Study the drawing (mm; zero at the part's minimum x, y, z) and answer. A direction names the side the tool comes from. Coordinates: 2 decimals unless noted, no trailing zeros. Order: outer loops, then holes, each group sorted by start corner. A loop starts at its lowest first (then second) coordinate and runs counter-clockwise, first axis right, second up. Notation, with made-up numbers: (-30, -18) -> (22, -18) arc R28 cw to (22, 11) -> close; hole circle Ø10 at (19.5, 55). An arc over 180 degrees is marked (long way). Answer as CSV lines item,"result". Start each with the question number.
Item 1: Each of these flat-tipped pins is pushed along its axis until it touches: pin 1 Ø4 at (x, y) = (15.5, 8) entering from -Z; pin 2 Ø1.5 at (x, y) = (18, 8) entering from +Z; pin 3 Ø5 at (x, y) = (51.5, 6.5) entering from -Z; pin 4 Ø5.5 at (x, y) = (83, 7) entering from +Z. Where does it stop, or does it pass through?
Item 2: Section B-B (y = 2.75) is taken. Write down the section's boundary in (x, z).
Item 3: For a pull along X with two mould halves and no side action, classify the marked faces 4 and 5 as pulls with the +X half, pulls with the -X half, needs draft (parallel to the pull), parting line crosses it, or undercut.
Item 4: Section A-A (z = 9) is taken. Write down the section's boundary in (x, y), then the cut area to 3 significant figures.
Item 5: Section D-D (z = 72.5) is taken. Write down the section's boundary in (x, y).
Item 6: Straight lines are drawn through the part: L1, parallel to X at y = 2, z = 95; L2, parallel to X at y = 9.75, z = 7.5; L3, parallel to Z at x = 62, y = 7.75. For each, find the intervals that lie inside material, in ascending order.
Item 7: Section C-C (x = 13) is taken. Write down the section's boundary in (y, z).
Item 8: Which of the six approach directions +Z, -Z, +X, -X, +Y, -Y give full straight-line access (tool end or side, diameter ignored) to the marked faces 1, 2 and 3?
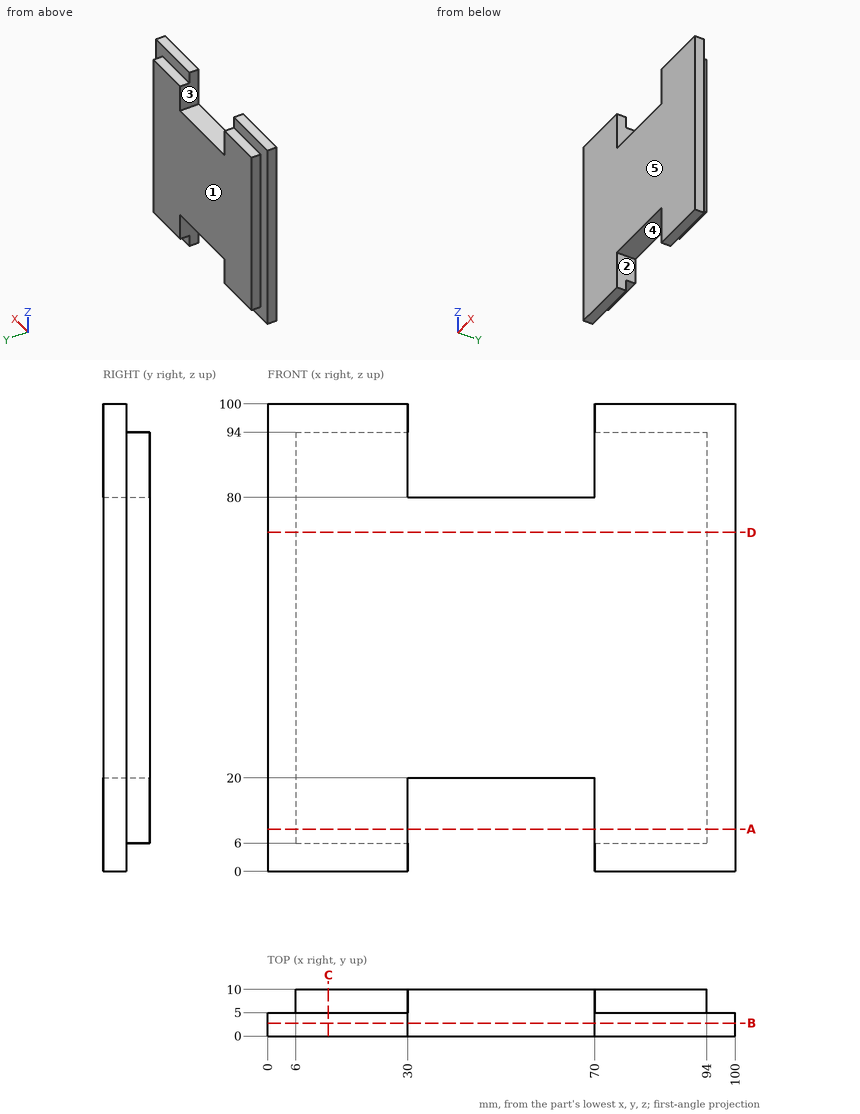
Checked values:
1,pin 1,"stops at z = 6"
1,pin 2,"stops at z = 94"
1,pin 3,"stops at z = 20"
1,pin 4,"stops at z = 100"
2,outline,"(0, 0) -> (30, 0) -> (30, 20) -> (70, 20) -> (70, 0) -> (100, 0) -> (100, 100) -> (70, 100) -> (70, 80) -> (30, 80) -> (30, 100) -> (0, 100) -> close"
3,face 4,"undercut"
3,face 5,"needs draft"
4,outline,"(0, 0) -> (30, 0) -> (30, 10) -> (6, 10) -> (6, 5) -> (0, 5) -> close; (70, 0) -> (100, 0) -> (100, 5) -> (94, 5) -> (94, 10) -> (70, 10) -> close"
4,area,"540 mm^2"
5,outline,"(0, 0) -> (100, 0) -> (100, 5) -> (94, 5) -> (94, 10) -> (6, 10) -> (6, 5) -> (0, 5) -> close"
6,L1,"x = 0 to 30, 70 to 100"
6,L2,"x = 6 to 30, 70 to 94"
6,L3,"z = 20 to 80"
7,outline,"(0, 0) -> (5, 0) -> (5, 6) -> (10, 6) -> (10, 94) -> (5, 94) -> (5, 100) -> (0, 100) -> close"
8,face 1,"+Z, -Z, +X, -X, +Y"
8,face 2,"-Z, +Y, -Y"
8,face 3,"+Z, +Y, -Y"
